Drawing for the job (mm, zero at the part's lowest x, y, z). Round coordinates to 2 decimals unless told otherwise and drop trailing zeros. Order: outer loops, then holes, each group sorted by start corner. A loop starts at its lowest first (then second) coordinate and runs counter-clockwise, first axis right, second up. Notation, with made-up numbers: (-35, 40.25) - (-31, 40.25) arc R22 cw to (-31, 63.25) - close; hole circle Ø6 at (25.5, 55). An arc over 180 degrees is marked (long way). Put each result on its own line as item: value. Start each with the question number.
Item 1: Probe probe 1 along Z at (x, y) = (1, 5.25); probe 2 along X at (y, z) = (6.25, 100.5); probe 3 along Y at (x, z) = (2, 39.5). List the from-to ranges inside material, lowest first.
Item 2: Saw through at C-C on z = 12.5. List the corners of the cut face in (x, y), plus the area to 3 significant figures.
Item 3: Saw through at A-A on y = 6. List the corners of the cut face in (x, z).
Item 4: Mould opens along Z. For the marked faces 1 and 2 say: pulls with the +Z half, pulls with the -Z half, needs draft (parallel to the pull), parting line crosses it, or undercut.
Item 5: Pin check, flat tips, straight feed: pin 1 Ø3 at (y, z) = (7, 89.5) entering from +X; pin 2 Ø6 at (x, z) = (9.5, 42.5) entering from +Y; pin 3 Ø2 at (x, z) = (10, 85) entering from -Y. Stop position of each tip, or through.
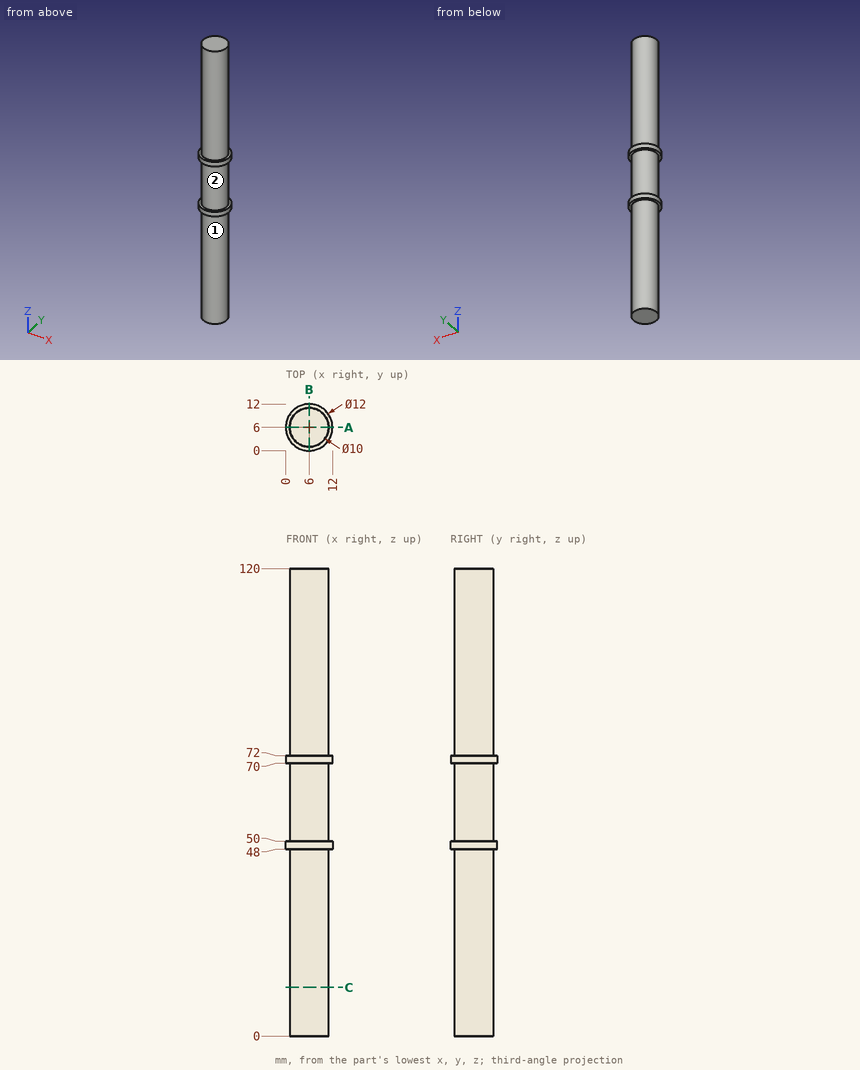
Results found:
1. probe 1: z = 48 to 50, 70 to 72
1. probe 2: x = 1.01 to 10.99
1. probe 3: y = 3 to 9
2. outline: circle Ø10 at (6, 6)
2. area: 78.5 mm²
3. outline: (0, 48) - (1, 48) - (1, 0) - (11, 0) - (11, 48) - (12, 48) - (12, 50) - (11, 50) - (11, 70) - (12, 70) - (12, 72) - (11, 72) - (11, 120) - (1, 120) - (1, 72) - (0, 72) - (0, 70) - (1, 70) - (1, 50) - (0, 50) - close
4. face 1: needs draft
4. face 2: undercut
5. pin 1: stops at x = 11
5. pin 2: stops at y = 10.97
5. pin 3: stops at y = 2
